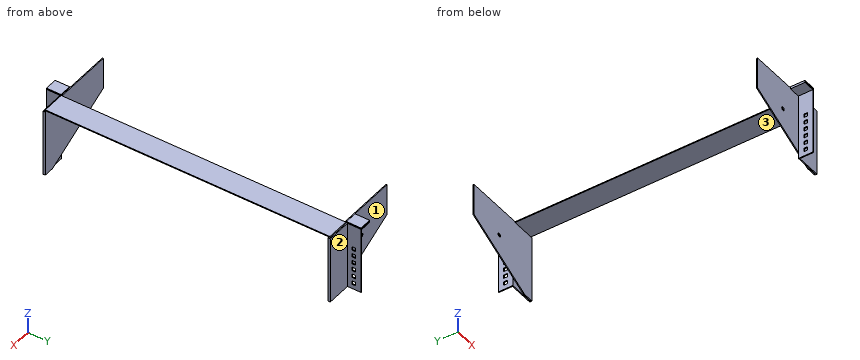
from build123d import *

# Parameters (mm, degrees)
F0_W      = 2
F0_H      = 148
F1_DEPTH  = 50
F3_DEPTH  = 130
F4_W      = 2
F4_H      = 148
F5_DEPTH  = 3
F6_W      = 2
F6_H      = 148
F7_DEPTH  = 5
F8_W      = 2
F8_H      = 148
F9_DEPTH  = 54
F10_W     = 2
F10_H     = 148
F11_DEPTH = 30
F13_DEPTH = 761
F14_W     = 2
F14_H     = 148
F15_DEPTH = 3
F16_W     = 2
F16_H     = 148
F17_DEPTH = 54
F18_W     = 2
F18_H     = 148
F19_DEPTH = 30
F20_W     = 32
F20_H     = 2
F21_DEPTH = 25
F22_W     = 2
F22_H     = 32
F23_DEPTH = 3
F24_W     = 32
F24_H     = 2
F25_DEPTH = 25
F26_W     = 8
F26_H     = 8
F27_DEPTH = 25
F28_W     = 32
F28_H     = 2
F29_DEPTH = 25
F30_W     = 2
F30_H     = 32
F31_DEPTH = 3
F32_W     = 32
F32_H     = 2
F33_DEPTH = 25
F34_W     = 8
F34_H     = 8
F35_DEPTH = 25
F37_D     = 8


with BuildPart() as f1:
    # F0 (on Right) → F1 (new body)
    with BuildSketch(Plane.YZ):
        Polygon((314, 150), (-314, 150), (-314, 148), (-312, 148), (312, 148), (314, 148), align=None)
        with Locations((313, 74)):
            Rectangle(F0_W, F0_H)
        with Locations((-313, 74)):
            Rectangle(F0_W, F0_H)
    extrude(amount=-F1_DEPTH)

    # F2 (on face) → F3 (join)
    with BuildSketch(Plane(origin=(-50, 0, 0), x_dir=(0, -1, 0), z_dir=(-1, 0, 0))):
        Polygon((312, 0), (314, 0), (314, 150), (312, 150), (312, 148), align=None)
        Polygon((-312, 0), (-312, 148), (-312, 150), (-314, 150), (-314, 0), align=None)
    extrude(amount=F3_DEPTH)

    # F4 (on face) → F5 (join)
    with BuildSketch(Plane.YZ):
        with Locations((313, 74)):
            Rectangle(F4_W, F4_H)
        with Locations((-313, 74)):
            Rectangle(F4_W, F4_H)
    extrude(amount=F5_DEPTH)

    # F6 (on face) → F7 (join)
    with BuildSketch(Plane(origin=(0, -312, 0), x_dir=(-1, 0, 0), z_dir=(0, 1, 0))):
        with Locations((-2, 74)):
            Rectangle(F6_W, F6_H)
    extrude(amount=-F7_DEPTH)

    # F8 (on face) → F9 (join)
    with BuildSketch(Plane(origin=(1, 0, 0), x_dir=(0, -1, 0), z_dir=(-1, 0, 0))):
        with Locations((316, 74)):
            Rectangle(F8_W, F8_H)
    extrude(amount=F9_DEPTH)

    # F10 (on face) → F11 (join)
    with BuildSketch(Plane.XZ.offset(317)):
        with Locations((-52, 74)):
            Rectangle(F10_W, F10_H)
    extrude(amount=F11_DEPTH)

    # F12 (on face) → F13 (cut)
    with BuildSketch(Plane.XZ.offset(314)):
        Polygon((-180, 0), (-20, 0), (-180, 80), align=None)
    extrude(amount=-F13_DEPTH, mode=Mode.SUBTRACT)

    # F14 (on face) → F15 (join)
    with BuildSketch(Plane(origin=(0, 314, 0), x_dir=(-1, 0, 0), z_dir=(0, 1, 0))):
        with Locations((-2, 74)):
            Rectangle(F14_W, F14_H)
    extrude(amount=F15_DEPTH)

    # F16 (on face) → F17 (join)
    with BuildSketch(Plane(origin=(1, 0, 0), x_dir=(0, -1, 0), z_dir=(-1, 0, 0))):
        with Locations((-316, 74)):
            Rectangle(F16_W, F16_H)
    extrude(amount=F17_DEPTH)

    # F18 (on face) → F19 (join)
    with BuildSketch(Plane(origin=(0, 317, 0), x_dir=(-1, 0, 0), z_dir=(0, 1, 0))):
        with Locations((52, 74)):
            Rectangle(F18_W, F18_H)
    extrude(amount=F19_DEPTH)

    # F20 (on face) → F21 (join)
    with BuildSketch(Plane(origin=(-53, 0, 0), x_dir=(0, -1, 0), z_dir=(-1, 0, 0))):
        with Locations((-331, 147)):
            Rectangle(F20_W, F20_H)
    extrude(amount=F21_DEPTH)

    # F22 (on face) → F23 (join)
    with BuildSketch(Plane.XY.offset(148)):
        with Locations((-77, 331)):
            Rectangle(F22_W, F22_H)
    extrude(amount=F23_DEPTH)

    # F24 (on face) → F25 (join)
    with BuildSketch(Plane.YZ.offset(-76)):
        with Locations((331, 150)):
            Rectangle(F24_W, F24_H)
    extrude(amount=F25_DEPTH)

    # F26 (on face) → F27 (cut)
    with BuildSketch(Plane(origin=(-53, 0, 0), x_dir=(0, -1, 0), z_dir=(-1, 0, 0))):
        with Locations((-331, 94)):
            Rectangle(F26_W, F26_H)
        with Locations((-331, 78)):
            Rectangle(F26_W, F26_H)
        with Locations((-331, 62)):
            Rectangle(F26_W, F26_H)
        with Locations((-331, 46)):
            Rectangle(F26_W, F26_H)
        with Locations((-331, 30)):
            Rectangle(F26_W, F26_H)
        with Locations((-331, 14)):
            Rectangle(F26_W, F26_H)
    extrude(amount=-F27_DEPTH, mode=Mode.SUBTRACT)

    # F28 (on face) → F29 (join)
    with BuildSketch(Plane(origin=(-53, 0, 0), x_dir=(0, -1, 0), z_dir=(-1, 0, 0))):
        with Locations((331, 147)):
            Rectangle(F28_W, F28_H)
    extrude(amount=F29_DEPTH)

    # F30 (on face) → F31 (join)
    with BuildSketch(Plane.XY.offset(148)):
        with Locations((-77, -331)):
            Rectangle(F30_W, F30_H)
    extrude(amount=F31_DEPTH)

    # F32 (on face) → F33 (join)
    with BuildSketch(Plane.YZ.offset(-76)):
        with Locations((-331, 150)):
            Rectangle(F32_W, F32_H)
    extrude(amount=F33_DEPTH)

    # F34 (on face) → F35 (cut)
    with BuildSketch(Plane(origin=(-53, 0, 0), x_dir=(0, -1, 0), z_dir=(-1, 0, 0))):
        with Locations((331, 78)):
            Rectangle(F34_W, F34_H)
        with Locations((331, 62)):
            Rectangle(F34_W, F34_H)
        with Locations((331, 46)):
            Rectangle(F34_W, F34_H)
        with Locations((331, 30)):
            Rectangle(F34_W, F34_H)
        with Locations((331, 14)):
            Rectangle(F34_W, F34_H)
        with Locations((331, 94)):
            Rectangle(F34_W, F34_H)
    extrude(amount=-F35_DEPTH, mode=Mode.SUBTRACT)

    # F37 (through all)
    with Locations(Plane.XZ.offset(314)):
        with Locations((-100, 85)):
            Hole(F37_D / 2)


solid = f1.part
Source: CAD feature listing. Evaluate the final solid. Frame: model axes, mm. Face numbers are marked on the shaded views. Round coordinates to 2 decimals unless told otherwise and drop trailing zeros. Loops run counter-clockwise (first coordinate to the right, second up) from the corner with the lowest first, then second, coordinate; pieces in that order, holes last. Notation, with made-up numbers: M -26.5,23 L 9.5,23 A18 ccw 9.5,50 Z; hole C 43,-21 d4. An arc over 180 degrees is marked long. Answer as CSV lines item,"result".
Q1. Cut plane A-A (x = -161.5). Return the cut outline in (y, z).
Verdict:
outline,"M -314,70.75 L -312,70.75 L -312,150 L -314,150 Z; M 312,70.75 L 314,70.75 L 314,150 L 312,150 Z"
Q2. Pull-direction query (Y, two-part tool) for the marked faces 1, 2 and 3; classes: +Y half, -Y half, draft (parallel to the pull), parting line (faces both ways), or undercut.
Verdict:
face 1,"undercut"
face 2,"+Y half"
face 3,"undercut"
Q3. Line query: line 1 along Y through (x, z) = (-41.5, 136); line 2 along Y through (x, z) = (-157.5, 136); line 3 along Z through (x, y) = (-100, 313). Output: solid intervals per line, ascending.
Verdict:
line 1,"y = -317 to -315, -314 to -312, 312 to 314, 315 to 317"
line 2,"y = -314 to -312, 312 to 314"
line 3,"z = 40 to 81, 89 to 150"
Q4. Contact query for flat-ended pins moving along their axis: pin 1 (9 mm diameter, centred on x = -100, z = 85, fed in from +Y); pin 2 (1 mm diameter, centred on y = -327, z = 149.5, fed in from +X); pin 3 (1 mm diameter, centred on x = -24, y = -100, fed in from +Z); pin 4 (10 mm diameter, centred on x = -98, z = 31.5, fed in from +Y) (3 decimals). Output: stop coordinate, or through.
Verdict:
pin 1,"stops at y = 314"
pin 2,"stops at x = -51"
pin 3,"stops at z = 150"
pin 4,"passes through"
Q5. Cut plane C-C (y = -266). Return the cut outline in (x, z).
Verdict:
outline,"M -50,148 L 0,148 L 0,150 L -50,150 Z"
Q6. Cut plane B-B (z = 109.5). Return the cut outline in (x, y).
Verdict:
outline,"M -180,-314 L 1,-314 L 1,-315 L -53,-315 L -53,-347 L -51,-347 L -51,-317 L 3,-317 L 3,-312 L -180,-312 Z; M -180,312 L 3,312 L 3,317 L -51,317 L -51,347 L -53,347 L -53,315 L 1,315 L 1,314 L -180,314 Z"
